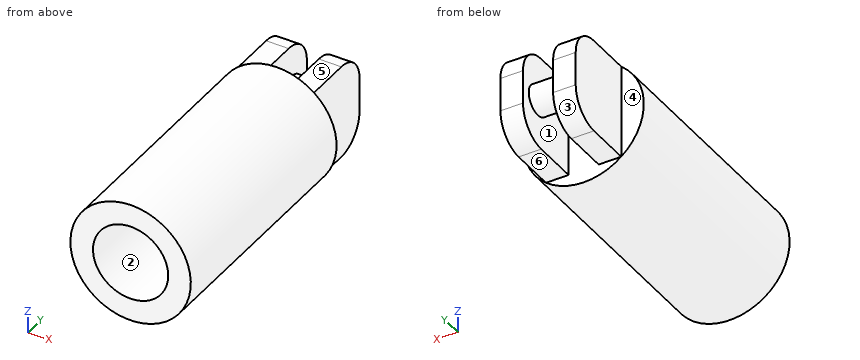
from build123d import *

# Parameters (mm, degrees)
SKETCH1_R           = 50.8
BOSS_EXTRUDE1_DEPTH = 203.2
SKETCH2_W           = 63.5
SKETCH2_H           = 79.31147458
BOSS_EXTRUDE2_DEPTH = 63.5
SKETCH3_W           = 25.4
SKETCH3_H           = 79.31147458
CUT_EXTRUDE1_DEPTH  = 63.5
FILLET1_R           = 25.4
SKETCH4_R           = 31.75
CUT_EXTRUDE2_DEPTH  = 63.5
SKETCH5_R           = 12.7
BOSS_EXTRUDE3_DEPTH = 53.34


with BuildPart() as part:
    # Sketch1 → Boss-Extrude1 (new body)
    with BuildSketch(Plane(origin=(0, 0, 0), x_dir=(1, 0, 0), z_dir=(0, 1, 0))):
        with Locations(Location((0, 0, 0), (0, 0, 270))):
            Circle(SKETCH1_R)
    extrude(amount=BOSS_EXTRUDE1_DEPTH)

    # Sketch2 → Boss-Extrude2 (add)
    with BuildSketch(Plane(origin=(0, 203.2, 0), x_dir=(1, 0, 0), z_dir=(0, 1, 0))):
        Rectangle(SKETCH2_W, SKETCH2_H)
    extrude(amount=BOSS_EXTRUDE2_DEPTH)

    # Sketch3 → Cut-Extrude1 (cut)
    with BuildSketch(Plane(origin=(0, 266.7, 0), x_dir=(1, 0, 0), z_dir=(0, 1, 0))):
        Rectangle(SKETCH3_W, SKETCH3_H)
    extrude(amount=-CUT_EXTRUDE1_DEPTH, mode=Mode.SUBTRACT)

    # Fillet1
    fillet1_edges = [part.edges().sort_by_distance(p)[0] for p in [
        (22.225, 266.7, -39.65573729),
        (-22.225, 266.7, 39.65573729),
        (-22.225, 266.7, -39.65573729),
        (22.225, 266.7, 39.65573729),
    ]]
    fillet(fillet1_edges, radius=FILLET1_R)

    # Sketch4 → Cut-Extrude2 (cut)
    with BuildSketch(Plane.XZ):
        with Locations(Location((0, 0, 0), (0, 0, 270))):
            Circle(SKETCH4_R)
    extrude(amount=-CUT_EXTRUDE2_DEPTH, mode=Mode.SUBTRACT)

    # Sketch5 → Boss-Extrude3 (add)
    with BuildSketch(Plane(origin=(31.75, 0, 0), x_dir=(0, 0, -1), z_dir=(1, 0, 0))):
        with Locations((0, 245.993497046)):
            Circle(SKETCH5_R)
    extrude(amount=-BOSS_EXTRUDE3_DEPTH)


solid = part.part
The listing builds one solid part. Answer for the finished solid, in the listing's coordinates (mm). Face numbers are marked on the shaded views. A direction names the side the tool comes from. Coordinates: 2 decimals unless noted, no trailing zeros. Write each loop counter-clockwise with the first axis right and the second up, starting at its lowest first coordinate (ties: lowest second). Pieces come first, ordered by that corner, then holes. Notation, with made-up numbers: M 47,53.25 L 103,53.25 A25 ccw 103,76.25 Z; hole C 70,41 d8. An arc over 180 degrees is marked long. Put each result on its own line as item: value. Start each with the question number.
1. A cutting plane is placed at D-D on y = 167. Write down the section's boundary in (x, z), then the cut area to 3 significant figures.
2. A cutting plane is placed at C-C on z = -35. Write down the section's boundary in (x, y).
3. Which of the six approach directions +Z, -Z, +X, -X, +Y, -Y give full straight-line access (tool end or side, diameter ignored) to the marked faces 4, 5 and 6?
4. Consider line 1 (X direction, y = 34.5, z = 0); line 2 (Y direction, x = -32, z = 9); line 3 (Y direction, x = 20, z = -8.5). Determine where each line is inside the solid, lowest interval first. Write a range as from..to.
5. A cutting plane is placed at A-A on z = 0. Write down the section's boundary in (x, y).
6. For a pull along Z with two mould halves and no side action, classify the marked faces 1, 2 and 3 as pulls with the +Z half, pulls with the -Z half, needs draft (parallel to the pull), parting line crosses it, or undercut.
7. A cutting plane is placed at B-B on x = -6.5. Write down the section's boundary in (y, z).
8. Flat-ended cylindrical pins translate along their axes: P1, Ø12, axis at x = -31, y = 65, coming from the +Z side; P2, Ø2, axis at y = 233, z = -24, coming from the -X side; P3, Ø9.5, axis at x = -25.5, y = 224, coming from the -Z side. Find the tip coordinate at first contact, or state that the pin passes through.
Resolved:
1. outline: C 0,0 d101.6
1. area: 8,110 mm2
2. outline: M -36.82,0 L 36.82,0 L 36.82,203.2 L 31.75,203.2 L 31.75,255.96 L 12.7,255.96 L 12.7,203.2 L -12.7,203.2 L -12.7,255.96 L -31.75,255.96 L -31.75,203.2 L -36.82,203.2 Z
3. face 4: +Z, -Z, -X, +Y
3. face 5: +Z, +X, -X, +Y
3. face 6: -Z, +X, -X, +Y
4. line 1: x = -50.8..-31.75, 31.75..50.8
4. line 2: y = 0..203.2
4. line 3: y = 63.5..266.7
5. outline: M -50.8,0 L -31.75,0 L -31.75,63.5 L 31.75,63.5 L 31.75,0 L 50.8,0 L 50.8,203.2 L 31.75,203.2 L 31.75,266.7 L 12.7,266.7 L 12.7,258.69 L -12.7,258.69 L -12.7,266.7 L -31.75,266.7 L -31.75,203.2 L -50.8,203.2 Z; hole M -12.7,203.2 L 12.7,203.2 L 12.7,233.29 L -12.7,233.29 Z
6. face 1: needs draft
6. face 2: undercut
6. face 3: pulls with the -Z half
7. outline: M 0,-50.38 L 203.2,-50.38 L 203.2,50.38 L 0,50.38 L 0,31.08 L 63.5,31.08 L 63.5,-31.08 L 0,-31.08 Z; C 245.99,0 d25.4
8. P1: stops at z = 44.22
8. P2: stops at x = -31.75
8. P3: stops at z = -39.66
